Geometry: final body of the model. Coordinates: model frame, mm. A direction names the side the tool comes from. Give positions to 0.01 mm unless a question says otherwise; leave off trailing zeros. Write each loop counter-clockwise with the first axis right and the second up, starting at its lowest first coordinate (ties: lowest second). Pieces come first, ordered by that corner, then holes. Notation, with made-up numbers: M 36,56 L 78,56 A23 ccw 78,79 Z; hole C 23,86 d6. An arc over 180 degrees is marked long. Answer as a JSON object with one key per item and string values.
from build123d import *

# Parameters (mm, degrees)
EXTRUDE_1_DEPTH     = 4
SKETCH_3_W          = 43.235473071
SKETCH_3_H          = 2
EXTRUDE_2_DEPTH     = 20
SKETCH_4_W          = 43.235473071
SKETCH_4_H          = 21
EXTRUDE_3_DEPTH     = 15
SKETCH_8_W          = 3
SKETCH_8_H          = 10
EXTRUDE_4_DEPTH     = 10
SKETCH_10_R         = 1.4
CUT_EXTRUDE_1_DEPTH = 83
SKETCH_11_W         = 3
SKETCH_11_H         = 90
EXTRUDE_5_DEPTH     = 80
SKETCH_12_W         = 75
SKETCH_12_H         = 25
EXTRUDE_6_DEPTH     = 5
SKETCH_13_W         = 23
SKETCH_13_H         = 20
CUT_EXTRUDE_2_DEPTH = 4
CUT_EXTRUDE_3_REACH = 123
SKETCH_14_W         = 7.5
SKETCH_14_H         = 5
SKETCH_15_R         = 1.1
CUT_EXTRUDE_4_DEPTH = 10
SKETCH_17_W         = 3
SKETCH_17_H         = 10
EXTRUDE_7_DEPTH     = 10
SKETCH_18_R         = 1.1
CUT_EXTRUDE_5_DEPTH = 3
SKETCH_19_W         = 3
SKETCH_19_H         = 10
EXTRUDE_8_DEPTH     = 10
SKETCH_20_R         = 1.1
CUT_EXTRUDE_6_DEPTH = 3


with BuildPart() as part:
    # 草圖1 → 填料-伸長1 (new body)
    with BuildSketch(Plane.XY):
        Polygon((-37.5, 45), (-35, 45), (-35, 80), (15, 80), (15, 45), (37.5, 45), (37.5, -45), (-37.5, -45), align=None)
    extrude(amount=EXTRUDE_1_DEPTH)

    # 草圖3 → 填料-伸長2 (add)
    with BuildSketch(Plane.XY.offset(4)):
        with Locations((-6.617736535, 56)):
            Rectangle(SKETCH_3_W, SKETCH_3_H)
        with Locations((-6.617736535, 79)):
            Rectangle(SKETCH_3_W, SKETCH_3_H)
    extrude(amount=EXTRUDE_2_DEPTH)

    # 草圖4 → 填料-伸長3 (add)
    with BuildSketch(Plane.XY.offset(4)):
        with Locations((-6.617736535, 67.5)):
            Rectangle(SKETCH_4_W, SKETCH_4_H)
    extrude(amount=EXTRUDE_3_DEPTH)

    # 草圖8 → 填料-伸長4 (add)
    with BuildSketch(Plane(origin=(0, 0, 0), x_dir=(-1, 0, 0), z_dir=(0, 0, -1))):
        with Locations((-36, 40)):
            Rectangle(SKETCH_8_W, SKETCH_8_H)
        with Locations((36, 40)):
            Rectangle(SKETCH_8_W, SKETCH_8_H)
        with Locations((36, -40)):
            Rectangle(SKETCH_8_W, SKETCH_8_H)
        with Locations((-36, -40)):
            Rectangle(SKETCH_8_W, SKETCH_8_H)
    extrude(amount=EXTRUDE_4_DEPTH)

    # 草圖10 → 除料-伸長1 (cut)
    with BuildSketch(Plane(origin=(37.5, 0, 0), x_dir=(0, 0, -1), z_dir=(1, 0, 0))):
        with Locations((5, 40)):
            Circle(SKETCH_10_R)
        with Locations((5, -40)):
            Circle(SKETCH_10_R)
    extrude(amount=-CUT_EXTRUDE_1_DEPTH, mode=Mode.SUBTRACT)

    # 草圖11 → 填料-伸長5 (add)
    with BuildSketch(Plane.XY.offset(4)):
        with Locations((36, 0)):
            Rectangle(SKETCH_11_W, SKETCH_11_H)
    extrude(amount=EXTRUDE_5_DEPTH)

    # 草圖12 → 填料-伸長6 (add)
    with BuildSketch(Plane.XZ.offset(45)):
        with Locations((0, 61.5)):
            Rectangle(SKETCH_12_W, SKETCH_12_H)
    extrude(amount=-EXTRUDE_6_DEPTH)

    # 草圖13 → 除料-伸長2 (cut)
    with BuildSketch(Plane.XZ.offset(45)):
        with Locations((-26, 64)):
            Rectangle(SKETCH_13_W, SKETCH_13_H)
    extrude(amount=-CUT_EXTRUDE_2_DEPTH, mode=Mode.SUBTRACT)

    # 草圖14 → 除料-伸長3 (cut, up to next)
    with BuildSketch(Plane.XZ.offset(41), mode=Mode.PRIVATE) as cut_extrude_3_sk1:
        with Locations((-33.75, 71.5)):
            Rectangle(SKETCH_14_W, SKETCH_14_H)
    cut_extrude_3_tool1 = extrude(cut_extrude_3_sk1.sketch, amount=-CUT_EXTRUDE_3_REACH, mode=Mode.PRIVATE) & part.part
    add(cut_extrude_3_tool1.solids().sort_by_distance((-33.75, -41, 71.5))[0], mode=Mode.SUBTRACT)

    # 草圖15 → 除料-伸長4 (cut)
    with BuildSketch(Plane(origin=(15, 0, 0), x_dir=(0, 0, -1), z_dir=(1, 0, 0))):
        with Locations((-16.1, 72.2)):
            Circle(SKETCH_15_R)
        with Locations((-16.1, 62.8)):
            Circle(SKETCH_15_R)
    extrude(amount=-CUT_EXTRUDE_4_DEPTH, mode=Mode.SUBTRACT)

    # 草圖17 → 填料-伸長7 (add)
    with BuildSketch(Plane.XY.offset(4)):
        with Locations((-36, 40)):
            Rectangle(SKETCH_17_W, SKETCH_17_H)
    extrude(amount=EXTRUDE_7_DEPTH)

    # 草圖18 → 除料-伸長5 (cut)
    with BuildSketch(Plane.ZY.offset(37.5)):
        with Locations((9, 40)):
            Circle(SKETCH_18_R)
    extrude(amount=-CUT_EXTRUDE_5_DEPTH, mode=Mode.SUBTRACT)

    # 草圖19 → 填料-伸長8 (add)
    with BuildSketch(Plane.XY.offset(4)):
        with Locations((-36, -40)):
            Rectangle(SKETCH_19_W, SKETCH_19_H)
    extrude(amount=EXTRUDE_8_DEPTH)

    # 草圖20 → 除料-伸長6 (cut)
    with BuildSketch(Plane.ZY.offset(37.5)):
        with Locations((9, -40)):
            Circle(SKETCH_20_R)
    extrude(amount=-CUT_EXTRUDE_6_DEPTH, mode=Mode.SUBTRACT)


with BuildPart() as body_2:
    # 鏡射1: mirrored copy
    add(part.part.mirror(Plane(origin=(37.5, 0, 4), x_dir=(0, 0, 1), z_dir=(1, 0, 0))))


solid = body_2.part
1) Pull-direction query (Y, two-part tool) for faces 6 (the flat face through (40, 45, 30)), 7 (the flat face through (111, -35, 9)), 8 (the flat face through (39, -35, -5)), 9 (the flat face through (111, 40, 14)); classes: pulls with the +Y half, pulls with the -Y half, needs draft (parallel to the pull), parting line crosses it, or undercut.
Geometry check:
{"face 6": "pulls with the +Y half", "face 7": "undercut", "face 8": "undercut", "face 9": "needs draft"}
2) Line query: line 1 (Y direction, x = 110, z = 9); line 2 (Y direction, x = 110.55, z = -5); line 3 (Y direction, x = 65, z = 16). Output: solid intervals per line, ascending. Write a range as from..to.
Geometry check:
{"line 1": "y = -45..-41.1, -38.9..-35, 35..38.9, 41.1..45", "line 2": "y = -45..-41.4, -38.6..-35, 35..38.6, 41.4..45", "line 3": "y = 55..61.7, 63.9..71.1, 73.3..80"}
3) Cut plane C-C on x = 54. Return loops of the section in (y, z), and give its area (3 significant figures).
Geometry check:
{"outline": "M -45,0 L 45,0 L 45,4 L -45,4 Z; M -45,49 L -40,49 L -40,74 L -45,74 Z", "area": "485 mm2"}
4) Cut plane D-D on z = 59. Return loops of the section in (x, y).
Geometry check:
{"outline": "M 37.5,-45 L 89.5,-45 L 89.5,-41 L 112.5,-41 L 112.5,-40 L 40.5,-40 L 40.5,45 L 37.5,45 Z"}
5) Cut plane A-A on x = 62. Return loops of the section in (y, z), and give its area (3 significant figures).
Geometry check:
{"outline": "M -45,0 L 80,0 L 80,24 L 78,24 L 78,19 L 57,19 L 57,24 L 55,24 L 55,4 L -45,4 Z; M -45,49 L -40,49 L -40,74 L -45,74 Z; hole C 62.8,16.1 d2.2; hole C 72.2,16.1 d2.2", "area": "1,010 mm2"}
6) Set-up query: faces 1 (the flat face through (82, 68, 19)), 2 (the flat face through (60, 66, 9)), 3 (the flat face through (66, -43, 74)), 4 (the flat face through (89.5, -43, 64)), 5 (the flat face through (39, 35, -5)). Return all of +Z, -Z, +X, -X, +Y, -Y with unobstructed straight access to the full face (end or side cutting, diameter ignored); none if empty.
Geometry check:
{"face 1": "+Z, +X, -X", "face 2": "+Z, -Z, -X, +Y", "face 3": "+Z, +X, +Y, -Y", "face 4": "+Z, +X, -Y", "face 5": "-Z, +X, -X"}
7) Contact query for flat-ended pins moving along their axis: P1, Ø4, axis at x = 66.5, y = -43.5, coming from the -Z side; P2, Ø2.5, axis at x = 75.5, y = -43, coming from the +Z side; P3, Ø12, axis at y = 56.5, z = 16, coming from the -X side. Output: stop coordinate, or through.
Geometry check:
{"P1": "stops at z = 0", "P2": "stops at z = 74", "P3": "stops at x = 60"}
8) Cut plane B-B on z = -5. Give the number of separate pieces and of enclosed holes in the cut face, and give its area (3 significant figures).
Geometry check:
{"separate pieces": "8", "enclosed holes": "0", "area": "86.4 mm2"}
